Input: part model. Units: mm. Frame: model coordinates. Give positions to 0.01 mm unless a question says otherwise; leave off trailing zeros. Write each loop counter-clockwise with the first axis right and the second up, starting at its lowest first coordinate (ties: lowest second). Pieces come first, ordered by that corner, then holes.
```python
from build123d import *

# Parameters (mm, degrees)
BOSS_EXTRUDE1_DEPTH = 1.5875
SKETCH2_R           = 1.905000001
SKETCH2_R_2         = 1.905000002
SKETCH2_R_3         = 2.159000002
SKETCH2_R_4         = 2.286
CUT_EXTRUDE1_DEPTH  = 69.454207549
CUT_EXTRUDE3_DEPTH  = 69.454207549
FILLET2_R           = 3.81


with BuildPart() as part:
    # Sketch1 → Boss-Extrude1 (new, symmetric)
    with BuildSketch(Plane(origin=(0, 0, 0), x_dir=(1, 0, 0), z_dir=(0, 1, 0))):
        Polygon((11.747500001, 20.002499998), (32.385000001, 43.179999998), (53.022500001, 20.002499998), (48.260000001, -8.172829969), (32.385000001, -2.857500002), (16.510000001, -8.172829969), align=None)
    extrude(amount=BOSS_EXTRUDE1_DEPTH, both=True)

    # Sketch2 → Cut-Extrude1 (cut, through all)
    with BuildSketch(Plane(origin=(0, -1.5875, 0), x_dir=(1, 0, 0), z_dir=(0, 1, 0))):
        with Locations(Location((19.684999998, 20.002500002, 0), (0, 0, 270))):
            Circle(SKETCH2_R)
        with Locations(Location((45.084999998, 20.0025, 0), (0, 0, 270))):
            Circle(SKETCH2_R_2)
        with Locations(Location((32.385000001, 34.925000025, 0), (0, 0, 270))):
            Circle(SKETCH2_R_3)
        with Locations(Location((23.747482722, 0.795511849, 0), (0, 0, 270))):
            Circle(SKETCH2_R_4)
        with Locations(Location((41.022517279, 0.795511849, 0), (0, 0, 90))):
            Circle(SKETCH2_R_4)
    extrude(amount=CUT_EXTRUDE1_DEPTH, mode=Mode.SUBTRACT)

    # Sketch4 → Cut-Extrude3 (cut, through all)
    with BuildSketch(Plane(origin=(0, 1.5875, 0), x_dir=(1, 0, 0), z_dir=(0, 1, 0))):
        Polygon((22.578091019, 16.887859433), (24.548137073, 5.232909805), (32.385000001, 7.856879088), (40.221862929, 5.232909805), (42.191908982, 16.887859433), (32.385000001, 27.901772597), align=None)
    extrude(amount=-CUT_EXTRUDE3_DEPTH, mode=Mode.SUBTRACT)

    # Fillet2
    fillet2_edges = [part.edges().sort_by_distance(p)[0] for p in [
        (53.022500001, 0, -20.002499998),
        (48.260000001, 0, 8.172829969),
        (32.385000001, 0, 2.857500002),
        (16.510000001, 0, 8.172829969),
        (11.747500001, 0, -20.002499998),
        (32.385000001, 0, -43.179999998),
        (22.578091019, 0, -16.887859433),
        (32.385000001, 0, -27.901772597),
        (42.191908982, 0, -16.887859433),
        (40.221862929, 0, -5.232909805),
        (32.385000001, 0, -7.856879088),
        (24.548137073, 0, -5.232909805),
    ]]
    fillet(fillet2_edges, radius=FILLET2_R)


solid = part.part
```
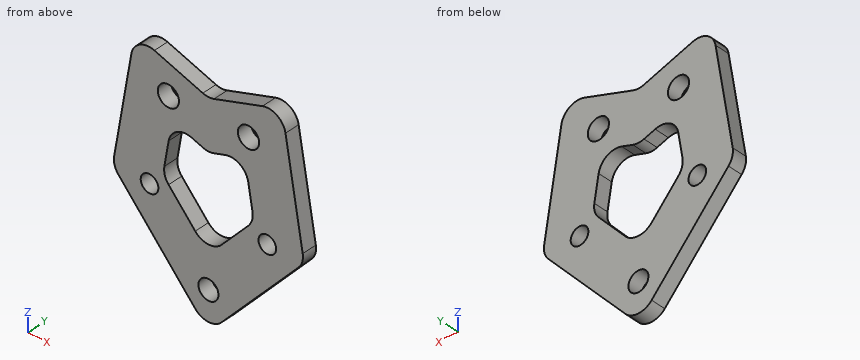
Q1. Section D-D, the plane x = 17. Return the cut outline in (y, z), then the cut area to 3 significant figures.
Q2. Pin query (flat end, axial travel): pin 1 (1.5 mm diameter, centred on x = 38.5, y = -1, fed in from -Z); pin 2 (4 mm diameter, centred on x = 46.5, z = -32.5, fed in from +Y); pin 3 (1 mm diameter, centred on y = 0, z = -20.5, fed in from -X); pin 4 (1 mm diameter, centred on y = -0.5, z = -20.5, fed in from +X). Return the tip coordinate at first contact, or that it passes through.
Q3. Section B-B, the plane y = 1.1. Give the number of separate pieces and of enclosed holes in the cut face, then the cut area to 3 significant figures.
Q4. Section C-C, the plane z = -27.5. Return the cut outline in (x, y).
Q5. Section A-A, the plane x = 46. Return the cut outline in (y, z), then the cut area to 3 significant figures.
Q6. Material intervals for line 1 along Z through (x, y) = (30.5, 0.8); line 2 along X through (y, z) = (0.5, -21.5); line 3 along Z through (x, y) = (31, -1.5), sorted ascending.
Solutions:
1. outline: (-1.59, -25.9) - (1.59, -25.9) - (1.59, 6) - (-1.59, 6) - close
1. area: 101 mm2
2. pin 1: stops at z = -37.15
2. pin 2: passes through
2. pin 3: stops at x = 12.18
2. pin 4: stops at x = 52.59
3. separate pieces: 1
3. enclosed holes: 6
3. area: 1,060 mm2
4. outline: (18.42, -1.59) - (46.35, -1.59) - (46.35, 1.59) - (18.42, 1.59) - close
5. outline: (-1.59, -27.89) - (1.59, -27.89) - (1.59, -21.67) - (-1.59, -21.67) - close; (-1.59, -18.33) - (1.59, -18.33) - (1.59, 6.88) - (-1.59, 6.88) - close
5. area: 99.8 mm2
6. line 1: z = -40.76 to -35.98, -33.87 to -25.48, -7.23 to 3.49
6. line 2: x = 13.08 to 18.51, 20.86 to 26.68, 38.09 to 43.91, 46.26 to 51.69
6. line 3: z = -41 to -36.58, -33.27 to -25.72, -7.39 to 3.32
